The model under review builds one solid part; all positions refer to its coordinate system, in mm. Coordinates: 2 decimals unless noted, no trailing zeros. Answer in a Markdown table with one row per item.
```python
from build123d import *

# Parameters (mm, degrees)
SKETCH2_R           = 5
SKETCH2_R_2         = 4
BOSS_EXTRUDE1_DEPTH = 10


with BuildPart() as part:
    # Sketch2 → Boss-Extrude1 (new body)
    with BuildSketch(Plane.XY):
        with BuildLine():
            Line((-175, 190), (175, 190))
            ThreePointArc((175, 190), (185.606601718, 185.606601718), (190, 175))
            Line((190, 175), (190, -175))
            ThreePointArc((190, -175), (185.606601718, -185.606601718), (175, -190))
            Line((175, -190), (-175, -190))
            ThreePointArc((-175, -190), (-185.606601718, -185.606601718), (-190, -175))
            Line((-190, -175), (-190, 175))
            ThreePointArc((-190, 175), (-185.606601718, 185.606601718), (-175, 190))
        make_face()
        with Locations((-175, 175)):
            Circle(SKETCH2_R, mode=Mode.SUBTRACT)
        with Locations((0, 175)):
            Circle(SKETCH2_R, mode=Mode.SUBTRACT)
        with Locations((175, 175)):
            Circle(SKETCH2_R, mode=Mode.SUBTRACT)
        with Locations((175, 0)):
            Circle(SKETCH2_R, mode=Mode.SUBTRACT)
        with Locations((-175, 0)):
            Circle(SKETCH2_R, mode=Mode.SUBTRACT)
        with Locations((-175, -175)):
            Circle(SKETCH2_R, mode=Mode.SUBTRACT)
        with Locations((0, -175)):
            Circle(SKETCH2_R, mode=Mode.SUBTRACT)
        with Locations((175, -175)):
            Circle(SKETCH2_R, mode=Mode.SUBTRACT)
        Circle(SKETCH2_R_2, mode=Mode.SUBTRACT)
    extrude(amount=BOSS_EXTRUDE1_DEPTH)


solid = part.part
```
Item 1: Mouldability with a two-part tool opening along Y and no side actions: class faces 1 (the face through (-0.651, -170.043, 4.93)), 2 (the face through (-40, 3, 10)), 3 (the face through (-2, 190, 5)), 4 (the face through (2, -190, 5)) as +Y half, -Y half, draft (parallel to the pull), parting line (faces both ways), or undercut.
Check values:
| item | result |
|---|---|
| face 1 | undercut |
| face 2 | draft |
| face 3 | +Y half |
| face 4 | -Y half |
Item 2: Clearance check with a flat-ended pin moving along its axis: pin 1 Ø6 at (x, y) = (0, -175) entering from +Z. State where the tip first meets the part, or that it passes through.
Check values:
| item | result |
|---|---|
| pin 1 | through |
Item 3: To check wall thickness, follow line 1 (Y direction, x = -175, z = 7); line 2 (Y direction, x = 0, z = 6.75). State the ranges of each line that lie inside material, in increasing order. Write a range as from..to.
Check values:
| item | result |
|---|---|
| line 1 | -190..-180, -170..-5, 5..170, 180..190 |
| line 2 | -190..-180, -170..-4, 4..170, 180..190 |
